Geometry check sheet. Reference: the model listing, model coordinates, mm. Face numbers are marked on the shaded views. A direction names the side the tool comes from. Round coordinates to 2 decimals unless told otherwise and drop trailing zeros. Loops run counter-clockwise (first coordinate to the right, second up) from the corner with the lowest first, then second, coordinate; pieces in that order, holes last.
```python
from build123d import *

# Parameters (mm, degrees)
SKETCH1_W           = 395
SKETCH1_H           = 700
BOSS_EXTRUDE1_DEPTH = 150
BOSS_EXTRUDE2_DEPTH = 1


with BuildPart() as part:
    # Sketch1 → Boss-Extrude1 (new body)
    with BuildSketch(Plane.XY):
        with BuildLine():
            Line((-400, 740), (5, 740))
            ThreePointArc((5, 740), (29.748737342, 729.748737342), (40, 705))
            Line((40, 705), (40, -5))
            ThreePointArc((40, -5), (29.748737342, -29.748737342), (5, -40))
            Line((5, -40), (-400, -40))
            ThreePointArc((-400, -40), (-424.748737342, -29.748737342), (-435, -5))
            Line((-435, -5), (-435, 705))
            ThreePointArc((-435, 705), (-424.748737342, 729.748737342), (-400, 740))
        make_face()
        with Locations((-197.5, 350)):
            Rectangle(SKETCH1_W, SKETCH1_H, mode=Mode.SUBTRACT)
    extrude(amount=BOSS_EXTRUDE1_DEPTH)

    # Sketch2 → Boss-Extrude2 (add)
    with BuildSketch(Plane.XY.offset(150)):
        with BuildLine():
            Line((-400, -40), (5, -40))
            ThreePointArc((5, -40), (29.748737342, -29.748737342), (40, -5))
            Line((40, -5), (40, 705))
            ThreePointArc((40, 705), (29.748737342, 729.748737342), (5, 740))
            Line((5, 740), (-400, 740))
            ThreePointArc((-400, 740), (-424.748737342, 729.748737342), (-435, 705))
            Line((-435, 705), (-435, -5))
            ThreePointArc((-435, -5), (-424.748737342, -29.748737342), (-400, -40))
        make_face()
    extrude(amount=BOSS_EXTRUDE2_DEPTH)


solid = part.part
```
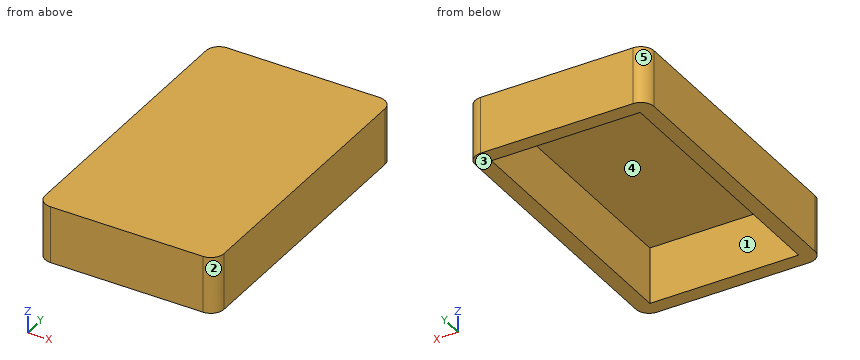
1) Mould release check, pull along X, two halves, no side actions. Record for the marked faces 1, 2 and 3: +X half, -X half, draft (parallel to the pull), parting line (faces both ways), or undercut.
Report:
face 1: undercut
face 2: +X half
face 3: draft
2) Sectioned sample at C-C, the plane x = -301. Record the cut outline in (y, z).
Report:
outline: (-40, 0) - (0, 0) - (0, 150) - (700, 150) - (700, 0) - (740, 0) - (740, 151) - (-40, 151) - close
3) Sectioned sample at B-B, the plane z = 79.5. Record the cut outline in (x, y), then the cut area to 3 significant figures.
Report:
outline: (-435, -5) arc R35 ccw to (-400, -40) - (5, -40) arc R35 ccw to (40, -5) - (40, 705) arc R35 ccw to (5, 740) - (-400, 740) arc R35 ccw to (-435, 705) - close; hole (-395, 0) - (0, 0) - (0, 700) - (-395, 700) - close
area: 92,900 mm2
4) Access from +Z, -Z, +X, -X, +Y, -Y to the whole of each face (thin tool, end or side, straight path). Record for the marked faces 4 and 5.
Report:
face 4: -Z
face 5: +Z, -Z, -X, +Y
5) Sectioned sample at A-A, the plane y = 369. Record the cut outline in (x, z).
Report:
outline: (-435, 0) - (-395, 0) - (-395, 150) - (0, 150) - (0, 0) - (40, 0) - (40, 151) - (-435, 151) - close
6) Scan lines: line 1 along Y through (x, z) = (-180.5, 75); line 2 along X through (y, z) = (241, 121); line 3 along Z through (x, y) = (-159, 273.5). Record each from-to range of solid material in increasing order.
Report:
line 1: y = -40 to 0, 700 to 740
line 2: x = -435 to -395, 0 to 40
line 3: z = 150 to 151
7) Gauge pin test, flat end, axial feed: pin 1 (2 mm diameter, centred on x = -237, y = 74, fed in from -Z). Record the tip position at first contact, or that the pin passes through.
Report:
pin 1: stops at z = 150
